Part model, mm, in its own coordinate system. Round coordinates to 2 decimals unless told otherwise and drop trailing zeros. Loops run counter-clockwise (first coordinate to the right, second up) from the corner with the lowest first, then second, coordinate; pieces in that order, holes last. Notation, with made-up numbers: (3.5, 50) - (51.5, 50) arc R19 cw to (51.5, 58) - close; hole circle Ø3 at (54.5, -12.5). An arc over 180 degrees is marked (long way). Put each result on its own line as item: value.
from build123d import *

# Parameters (mm, degrees)
F0_R     = 85
F1_DEPTH = 3


with BuildPart() as f1:
    # F0 (on Top) → F1 (new body)
    with BuildSketch(Plane.XY):
        with BuildLine():
            Line((90, 1.5), (94.988157, 1.5))
            ThreePointArc((94.988157, 1.5), (93.174602, 18.533581), (88.331639, 34.964575))
            Line((88.331639, 34.964575), (83.723183, 33.05569))
            Line((83.723183, 33.05569), (82.575133, 35.827328))
            Line((82.575133, 35.827328), (87.183589, 37.736213))
            ThreePointArc((87.183589, 37.736213), (78.989613, 52.779172), (68.22743, 66.10611))
            Line((68.22743, 66.10611), (64.70027, 62.57895))
            Line((64.70027, 62.57895), (62.57895, 64.70027))
            Line((62.57895, 64.70027), (66.10611, 68.22743))
            ThreePointArc((66.10611, 68.22743), (52.779172, 78.989613), (37.736213, 87.183589))
            Line((37.736213, 87.183589), (35.827328, 82.575133))
            Line((35.827328, 82.575133), (33.05569, 83.723183))
            Line((33.05569, 83.723183), (34.964575, 88.331639))
            ThreePointArc((34.964575, 88.331639), (18.533581, 93.174602), (1.5, 94.988157))
            Line((1.5, 94.988157), (1.5, 90))
            Line((1.5, 90), (-1.5, 90))
            Line((-1.5, 90), (-1.5, 94.988157))
            ThreePointArc((-1.5, 94.988157), (-18.533581, 93.174602), (-34.964575, 88.331639))
            Line((-34.964575, 88.331639), (-33.05569, 83.723183))
            Line((-33.05569, 83.723183), (-35.827328, 82.575133))
            Line((-35.827328, 82.575133), (-37.736213, 87.183589))
            ThreePointArc((-37.736213, 87.183589), (-52.779172, 78.989613), (-66.10611, 68.22743))
            Line((-66.10611, 68.22743), (-62.57895, 64.70027))
            Line((-62.57895, 64.70027), (-64.70027, 62.57895))
            Line((-64.70027, 62.57895), (-68.22743, 66.10611))
            ThreePointArc((-68.22743, 66.10611), (-78.989613, 52.779172), (-87.183589, 37.736213))
            Line((-87.183589, 37.736213), (-82.575133, 35.827328))
            Line((-82.575133, 35.827328), (-83.723183, 33.05569))
            Line((-83.723183, 33.05569), (-88.331639, 34.964575))
            ThreePointArc((-88.331639, 34.964575), (-93.174602, 18.533581), (-94.988157, 1.5))
            Line((-94.988157, 1.5), (-90, 1.5))
            Line((-90, 1.5), (-90, -1.5))
            Line((-90, -1.5), (-94.988157, -1.5))
            ThreePointArc((-94.988157, -1.5), (-93.174602, -18.533581), (-88.331639, -34.964575))
            Line((-88.331639, -34.964575), (-83.723183, -33.05569))
            Line((-83.723183, -33.05569), (-82.575133, -35.827328))
            Line((-82.575133, -35.827328), (-87.183589, -37.736213))
            ThreePointArc((-87.183589, -37.736213), (-78.989613, -52.779172), (-68.22743, -66.10611))
            Line((-68.22743, -66.10611), (-64.70027, -62.57895))
            Line((-64.70027, -62.57895), (-62.57895, -64.70027))
            Line((-62.57895, -64.70027), (-66.10611, -68.22743))
            ThreePointArc((-66.10611, -68.22743), (-52.779172, -78.989613), (-37.736213, -87.183589))
            Line((-37.736213, -87.183589), (-35.827328, -82.575133))
            Line((-35.827328, -82.575133), (-33.05569, -83.723183))
            Line((-33.05569, -83.723183), (-34.964575, -88.331639))
            ThreePointArc((-34.964575, -88.331639), (-18.533581, -93.174602), (-1.5, -94.988157))
            Line((-1.5, -94.988157), (-1.5, -90))
            Line((-1.5, -90), (1.5, -90))
            Line((1.5, -90), (1.5, -94.988157))
            ThreePointArc((1.5, -94.988157), (18.533581, -93.174602), (34.964575, -88.331639))
            Line((34.964575, -88.331639), (33.05569, -83.723183))
            Line((33.05569, -83.723183), (35.827328, -82.575133))
            Line((35.827328, -82.575133), (37.736213, -87.183589))
            ThreePointArc((37.736213, -87.183589), (52.779172, -78.989613), (66.10611, -68.22743))
            Line((66.10611, -68.22743), (62.57895, -64.70027))
            Line((62.57895, -64.70027), (64.70027, -62.57895))
            Line((64.70027, -62.57895), (68.22743, -66.10611))
            ThreePointArc((68.22743, -66.10611), (78.989613, -52.779172), (87.183589, -37.736213))
            Line((87.183589, -37.736213), (82.575133, -35.827328))
            Line((82.575133, -35.827328), (83.723183, -33.05569))
            Line((83.723183, -33.05569), (88.331639, -34.964575))
            ThreePointArc((88.331639, -34.964575), (93.174602, -18.533581), (94.988157, -1.5))
            Line((94.988157, -1.5), (90, -1.5))
            Line((90, -1.5), (90, 1.5))
        make_face()
        Circle(F0_R, mode=Mode.SUBTRACT)
    extrude(amount=F1_DEPTH)


solid = f1.part
1. Band-saw the part on B-B (x = 41.5). List the corners of the cut face in (y, z).
A:
outline: (-85.46, 0) - (-74.18, 0) - (-74.18, 3) - (-85.46, 3) - close; (74.18, 0) - (85.46, 0) - (85.46, 3) - (74.18, 3) - close
2. Two-plate mould, pull along Y, no slides. Class faces 1 (the cylindrical face through (-18.3, 93.22, 1.48)), 2 (the cylindrical face through (-67.453, -51.721, 1.479)), 3 (the cylindrical face through (-79.12, -52.58, 1.48)): pulls with the +Y half, pulls with the -Y half, needs draft (parallel to the pull), parting line crosses it, or undercut.
A:
face 1: pulls with the +Y half
face 2: undercut
face 3: pulls with the -Y half
3. Band-saw the part on A-A (y = 9). List the corners of the cut face in (x, z).
A:
outline: (-94.57, 0) - (-84.52, 0) - (-84.52, 3) - (-94.57, 3) - close; (84.52, 0) - (94.57, 0) - (94.57, 3) - (84.52, 3) - close
4. Probe line 1 along Y through (x, z) = (0, 1.25); line 2 along Y through (x, z) = (33.5, 2.4); line 3 along X through (y, z) = (-58.5, 2.5). List the from-to ranges inside material, lowest first. Write a range as [from, to].
A:
line 1: y = [-90, -85], [85, 90]
line 2: y = [-88.9, -84.8], [-83.54, -78.12], [78.12, 83.54], [84.8, 88.9]
line 3: x = [-74.85, -61.67], [61.67, 74.85]
5. Pin check, flat tips, straight feed: P1, Ø0.9, axis at x = -0.5, z = 1.5, coming from the +Y side; P2, Ø1, axis at y = 45, z = 1, coming from the +X side; P3, Ø1.5, axis at y = 18, z = 1, coming from the +X side. Stop position of each tip, or through.
A:
P1: stops at y = 90
P2: stops at x = 83.93
P3: stops at x = 93.42
